```python
from build123d import *

# Parameters (mm, degrees)
BOSS_EXTRUDE1_START = -5
SKETCH2_R           = 1.75
BOSS_EXTRUDE1_DEPTH = 5
FILLET1_R           = 1


with BuildPart() as part:
    # Sketch1 → Revolve1 (revolve)
    with BuildSketch(Plane.XY, mode=Mode.PRIVATE) as revolve1_sk:
        Polygon((-11.5, 0), (-16, 0), (-16, 1), (-12.5, 1), (-12.5, 41), (-12, 41), (-12, 39), (-11.5, 39), align=None)
    revolve(revolve1_sk.sketch.rotate(Axis((0, 0, 0), (0, 1, 0)), 270), axis=Axis((0, 0, 0), (0, 1, 0)))

    # Sketch2 → Boss-Extrude1 (add)
    # profile 1 of 2: a face of its own
    with BuildSketch(Plane.XZ.offset(BOSS_EXTRUDE1_START)):
        with BuildLine():
            Line((20.133991732, -9.046001908), (14.917336297, -5.785592261))
            ThreePointArc((14.917336297, -5.785592261), (13.567972864, -8.47998304), (11.737342657, -10.873582085))
            Line((11.737342657, -10.873582085), (16.953998092, -14.133991732))
            Line((16.953998092, -14.133991732), (20.133991732, -9.046001908))
        make_face()
        with Locations(Location((16, -10, 0), (0, 0, 270))):
            Circle(SKETCH2_R, mode=Mode.SUBTRACT)
    # profile 2 of 2: a face of its own
    with BuildSketch(Plane.XZ.offset(BOSS_EXTRUDE1_START)):
        with BuildLine():
            Line((-20.233087103, 9.715441438), (-15.116447525, 5.243378132))
            ThreePointArc((-15.116447525, 5.243378132), (-13.836527765, 8.034332543), (-12.047055108, 10.529409443))
            Line((-12.047055108, 10.529409443), (-16.284558562, 14.233087103))
            Line((-16.284558562, 14.233087103), (-20.233087103, 9.715441438))
        make_face()
        with Locations(Location((-16, 10, 0), (0, 0, 270))):
            Circle(SKETCH2_R, mode=Mode.SUBTRACT)
    extrude(amount=BOSS_EXTRUDE1_DEPTH)

    # Fillet1
    fillet1_edges = [part.edges().sort_by_distance(p)[0] for p in [
        (-20.233087103, 2.5, 9.715441438),
        (-16.284558562, 2.5, 14.233087103),
        (16.953998092, 2.5, -14.133991732),
        (20.133991732, 2.5, -9.046001908),
    ]]
    fillet(fillet1_edges, radius=FILLET1_R)


solid = part.part
```
Work out the finished part from the listing and answer in its coordinate system (mm). A direction names the side the tool comes from. Give positions to 0.01 mm unless a question says otherwise; leave off trailing zeros. Loops run counter-clockwise (first coordinate to the right, second up) from the corner with the lowest first, then second, coordinate; pieces in that order, holes last. Notation, with made-up numbers: (2.5, -11) -> (35.5, -11) arc R8 cw to (35.5, 1) -> close; hole circle Ø5 at (40, 41). An arc over 180 degrees is marked (long way). Write item = value, one per line. Start each with the question number.
(1) Find section B-B on x = 0. Give the vertices of the cut face in (y, z), and give its area (3 significant figures).
(2) Given pin 1 Ø4.5 at (x, z) = (16, -10) entering from +Y; pin 2 Ø5 at (x, z) = (15, 8) entering from -Y; pin 3 Ø2 at (x, y) = (-10, 13.5) entering from +Z; pin 4 Ø1 at (x, y) = (-7, 35.5) entering from -Z, each flat-ended and moving along its own axis, determine where each tip first touches the part or whether it passes through.
(3) Which of the six approach directions +Z, -Z, +X, -X, +Y, -Y give full straight-line access (tool end or side, diameter ignored) to faces 4 (the cylindrical face through (19.73, 2.46, -9.13)), 5 (the flat face through (13.89, 2.54, -12.22)), 6 (the flat face through (8, 1, 10)), 7 (the flat face through (-13.765, 2.535, 12.031))?
(4) Find section C-C on y = 11.5. Give the vertices of the cut face in (x, z), and give its area (3 significant figures).
(5) Find the intervals of material crossed by probe 1 along X at (y, z) = (39.75, 0); probe 2 along X at (y, z) = (2.15, -10); probe 3 along Y at (x, z) = (-4, 13), in increasing order. Write a range as from..to.
(6) The mould has two halves that part along X. Classify faces 1 (the flat face through (17.13, 2.54, -7.17)), 2 (the flat face through (-17.33, 2.54, 7.18)), 3 (the cylindrical face through (-9.7, 19.23, -6.18)): +X half, -X half, draft (parallel to the pull), parting line (faces both ways), or undercut.
(7) Find section A-A on z = 0. Give the vertices of the cut face in (x, y).
From the geometry:
q1.outline = (0, -16) -> (1, -16) -> (1, -12.5) -> (41, -12.5) -> (41, -12) -> (39, -12) -> (39, -11.5) -> (0, -11.5) -> close; (0, 11.5) -> (39, 11.5) -> (39, 12) -> (41, 12) -> (41, 12.5) -> (1, 12.5) -> (1, 16) -> (0, 16) -> close
q1.area = 87.0 mm^2
q2.pin_1 = 5
q2.pin_2 = 0
q2.pin_3 = 8.67
q2.pin_4 = -10.68
q3.face_4 = +X, +Y, -Y
q3.face_5 = -Z, +Y, -Y
q3.face_6 = +Y
q3.face_7 = +Z, +Y, -Y
q4.outline = circle Ø25 at (0, 0); hole circle Ø23 at (0, 0)
q4.area = 75.4 mm^2
q5.probe_1 = -12.5..-12, 12..12.5
q5.probe_2 = -7.5..-5.68, 5.68..7.5, 12.49..14.25, 17.75..19.54
q5.probe_3 = 0..1
q6.face_1 = +X half
q6.face_2 = -X half
q6.face_3 = undercut
q7.outline = (-16, 0) -> (-11.5, 0) -> (-11.5, 39) -> (-12, 39) -> (-12, 41) -> (-12.5, 41) -> (-12.5, 1) -> (-16, 1) -> close; (11.5, 0) -> (16, 0) -> (16, 1) -> (12.5, 1) -> (12.5, 41) -> (12, 41) -> (12, 39) -> (11.5, 39) -> close
